The listing builds one solid part. Answer for the finished solid, in the listing's coordinates (mm). Coordinates: 2 decimals unless noted, no trailing zeros. Write each loop counter-clockwise with the first axis right and the second up, starting at its lowest first coordinate (ties: lowest second). Pieces come first, ordered by that corner, then holes. Notation, with made-up numbers: M 24,69 L 64,69 A10 cw 64,86 Z; hole C 9,37.5 d6. An arc over 180 degrees is marked long. Write item = value, one per line. Start each with the question number.
```python
from build123d import *

# Parameters (mm, degrees)
SKETCH1_W           = 100
SKETCH1_H           = 100
BOSS_EXTRUDE1_DEPTH = 5
SKETCH2_W           = 42
SKETCH2_H           = 42
CUT_EXTRUDE1_DEPTH  = 2
SKETCH3_R           = 5
CUT_EXTRUDE2_DEPTH  = 5


with BuildPart() as part:
    # Sketch1 → Boss-Extrude1 (new body)
    with BuildSketch(Plane(origin=(0, 0, 0), x_dir=(1, 0, 0), z_dir=(0, 1, 0))):
        Rectangle(SKETCH1_W, SKETCH1_H)
    extrude(amount=BOSS_EXTRUDE1_DEPTH)

    # Sketch2 → Cut-Extrude1 (cut)
    with BuildSketch(Plane(origin=(0, 5, 0), x_dir=(1, 0, 0), z_dir=(0, 1, 0))):
        with Locations((0, -29)):
            Rectangle(SKETCH2_W, SKETCH2_H)
    extrude(amount=-CUT_EXTRUDE1_DEPTH, mode=Mode.SUBTRACT)

    # Sketch3 → Cut-Extrude2 (cut)
    with BuildSketch(Plane(origin=(0, 5, 0), x_dir=(1, 0, 0), z_dir=(0, 1, 0))):
        with Locations(Location((-35, -25, 0), (0, 0, 270))):
            Circle(SKETCH3_R)
        with Locations(Location((35, -25, 0), (0, 0, 270))):
            Circle(SKETCH3_R)
        with Locations(Location((0, 35, 0), (0, 0, 270))):
            Circle(SKETCH3_R)
    extrude(amount=-CUT_EXTRUDE2_DEPTH, mode=Mode.SUBTRACT)


solid = part.part
```
1. The part is cut by section D-D, the plane z = 32. Write down the section's boundary in (x, y), and give its area (3 significant figures).
2. Straight lines are drawn through the part: L1, parallel to X at y = 3.85, z = 25; L2, parallel to X at y = 3.4, z = 40.5; L3, parallel to X at y = 1.1, z = 25. For each, find the intervals that lie inside material, in ascending order. Write a range as [from, to].
3. The part is cut by section B-B, the plane x = 35. Write down the section's boundary in (y, z), and give its area (3 significant figures).
4. For a pull along X with two mould halves and no side action, classify faces 1 (the face through (-50, 2, 1)), 2 (the face through (0, 3, 29)), 3 (the face through (-1, 5, -1)), 4 (the face through (50, 2, 1)) as pulls with the +X half, pulls with the -X half, needs draft (parallel to the pull), parting line crosses it, or undercut.
5. The part is cut by section A-A, the plane z = -35. Write down the section's boundary in (x, y), and give its area (3 significant figures).
6. Each of these flat-tipped pins is pushed along its axis until it touches: pin 1 (16 mm diameter, centred on x = 35, z = 25, fed in from -Y); pin 2 (0.6 mm diameter, centred on x = 2, y = 4, fed in from +Z); pin 3 (1 mm diameter, centred on x = -3, z = 35.5, fed in from +Y); pin 4 (8 mm diameter, centred on x = 0, z = -35, fed in from -Y). Where does it stop, or does it pass through?
7. The part is cut by section C-C, the plane y = 4.15. Write down the section's boundary in (x, z).
Solution:
q1.outline = M -50,0 L 50,0 L 50,5 L 21,5 L 21,3 L -21,3 L -21,5 L -50,5 Z
q1.area = 416 mm^2
q2.L1 = [-50, -40], [-30, -21], [21, 30], [40, 50]
q2.L2 = [-50, -21], [21, 50]
q2.L3 = [-50, -40], [-30, 30], [40, 50]
q3.outline = M 0,-50 L 5,-50 L 5,20 L 0,20 Z; M 0,30 L 5,30 L 5,50 L 0,50 Z
q3.area = 450 mm^2
q4.face_1 = pulls with the -X half
q4.face_2 = undercut
q4.face_3 = needs draft
q4.face_4 = pulls with the +X half
q5.outline = M -50,0 L -5,0 L -5,5 L -50,5 Z; M 5,0 L 50,0 L 50,5 L 5,5 Z
q5.area = 450 mm^2
q6.pin_1 = 0
q6.pin_2 = 8
q6.pin_3 = 3
q6.pin_4 = through
q7.outline = M -50,-50 L 50,-50 L 50,50 L 21,50 L 21,8 L -21,8 L -21,50 L -50,50 Z; hole C -35,25 d10; hole C 0,-35 d10; hole C 35,25 d10
